Verification items for this drawing (mm, ordinates from the low corner). A direction names the side the tool comes from. Round coordinates to 2 decimals unless told otherwise and drop trailing zeros.
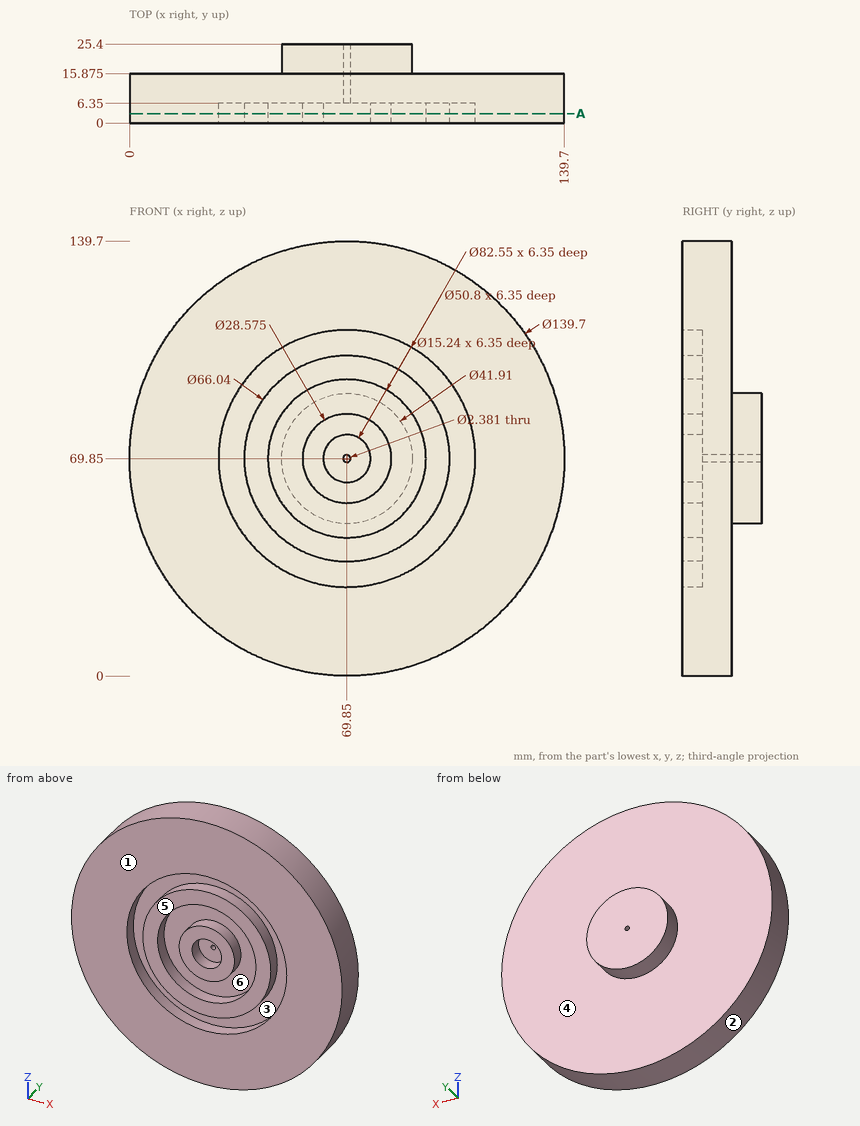
1. Depth check by flat-ended pin: pin 1 Ø10 at (x, y) = (67, 6.5) entering from -Z; pin 2 Ø6 at (x, z) = (111, 125.5) entering from -Y; pin 3 Ø10 at (y, z) = (12.5, 87) entering from -X (1 decimal); pin 4 Ø1.5 at (x, y) = (92, 8) entering from -Z. Enter the tip coordinate at first touch or a pass-through.
2. Release check for a two-part mould opening along Z. For the marked faces 1, 2 and 3 record: +Z half, -Z half, draft (parallel to the pull), parting line (faces both ways), or undercut.
3. Access from +Z, -Z, +X, -X, +Y, -Y to the whole of each face (thin tool, end or side, straight path). Record for the marked faces 4, 5 and 6.
4. Scan lines: line 1 along Z through (x, y) = (69.85, 12); line 2 along Z through (x, y) = (69.85, 19.75) (1 decimal). Record each from-to range of solid material in increasing order.
5. Section check A-A (y = 3). State how many separate pieces and enclosed holes the cut face has, plus the area to 3 significant figures.
Results below:
1. pin 1: stops at z = 0
1. pin 2: stops at y = 0
1. pin 3: stops at x = 1.1
1. pin 4: stops at z = 3.36
2. face 1: draft
2. face 2: parting line
2. face 3: undercut
3. face 4: +Y
3. face 5: +Z, -Z, +X, -X, -Y
3. face 6: -Y
4. line 1: z = 0 to 68.66, 71.04 to 139.7
4. line 2: z = 48.9 to 68.7, 71 to 90.8
5. separate pieces: 3
5. enclosed holes: 3
5. area: 11,800 mm2
